Check sheet for the modelled part. Datum: model origin and axes. Units: mm. Face numbers are marked on the shaded views. A direction names the side the tool comes from. Give positions to 0.01 mm unless a question says otherwise; leave off trailing zeros. Write each loop counter-clockwise with the first axis right and the second up, starting at its lowest first coordinate (ties: lowest second). Pieces come first, ordered by that corner, then holes. Notation, with made-up numbers: (-16.5, 43) -> (10.5, 43) arc R38 cw to (10.5, 82) -> close; hole circle Ø6 at (29.25, -2.5). An arc over 180 degrees is marked (long way). Use a Markdown table: item, result. Add a question column.
1. Cross-section at D-D (y = 32). Enter the section's corners in (x, z).
2. Cross-section at B-B (x = 73.5). Enter the section's corners in (y, z).
3. Scan lines: probe 1 along X at (y, z) = (23.5, -68); probe 2 along Y at (x, z) = (76, -69); probe 3 along Y at (x, z) = (64, -63). Record each from-to range of solid material in increasing order. Write a range as [from, to].
4. Cross-section at C-C (z = -65). Enter the section's corners in (x, y).
5. Cross-section at A-A (y = 58). Enter the section's corners in (x, z), then the cut area to 3 significant figures.
6. Gauge pin test, flat ends, axial feed: P1, Ø12, axis at x = 43, z = -59.5, coming from the +Y side; P2, Ø5, axis at x = 86, y = 21, coming from the +Z side; P3, Ø12.5, axis at x = 12.5, y = 51.5, coming from the -Z side. Record the tip position at first contact, or that the pin passes through.
7. Set-up check for the marked faces 1, 2, 3 and 4: record each of +Z, -Z, +X, -X, +Y, -Y from which the full face is reachable in a straight line by a thin tool's end or side.
8. Release check for a two-part mould opening along Y. For the marked faces 5, 6 and 7 record: released by +Y, released by -Y, zero draft, split by the parting line, or undercut.
from build123d import *

# Parameters (mm, degrees)
BOSS_EXTRUDE1_DEPTH = 40
SKETCH1_3_W         = 50
SKETCH1_3_H         = 40
BOSS_EXTRUDE2_DEPTH = 20
BOSS_EXTRUDE3_DEPTH = 65
SKETCH2_W           = 10
SKETCH2_H           = 41
CUT_EXTRUDE1_DEPTH  = 141.890028036


with BuildPart() as part:
    # Sketch1 → Boss-Extrude1 (new body)
    with BuildSketch(Plane(origin=(0, 0, 0), x_dir=(1, 0, 0), z_dir=(0, 1, 0))):
        Polygon((0, 75), (0, 25), (30, 25), (30, 10), (70, 10), (70, 25), (100, 25), (100, 75), (75, 75), (75, 35), (25, 35), (25, 75), align=None)
    extrude(amount=BOSS_EXTRUDE1_DEPTH)

    # Sketch1_3 → Boss-Extrude2 (add)
    with BuildSketch(Plane(origin=(0, 0, 0), x_dir=(1, 0, 0), z_dir=(0, 1, 0))):
        with Locations((50, 55)):
            Rectangle(SKETCH1_3_W, SKETCH1_3_H)
    extrude(amount=BOSS_EXTRUDE2_DEPTH)

    # Sketch1_4 → Boss-Extrude3 (add)
    with BuildSketch(Plane(origin=(0, 0, 0), x_dir=(1, 0, 0), z_dir=(0, 1, 0))):
        Polygon((70, 25), (70, 10), (70, 0), (100, 0), (100, 25), align=None)
        Polygon((0, 25), (0, 0), (30, 0), (30, 10), (30, 25), align=None)
    extrude(amount=BOSS_EXTRUDE3_DEPTH)

    # Sketch2 → Cut-Extrude1 (cut, through all)
    with BuildSketch(Plane(origin=(100, 0, 0), x_dir=(0, 0, -1), z_dir=(1, 0, 0))):
        with Locations((5, 32.5)):
            Rectangle(SKETCH2_W, SKETCH2_H)
    extrude(amount=-CUT_EXTRUDE1_DEPTH, mode=Mode.SUBTRACT)


solid = part.part
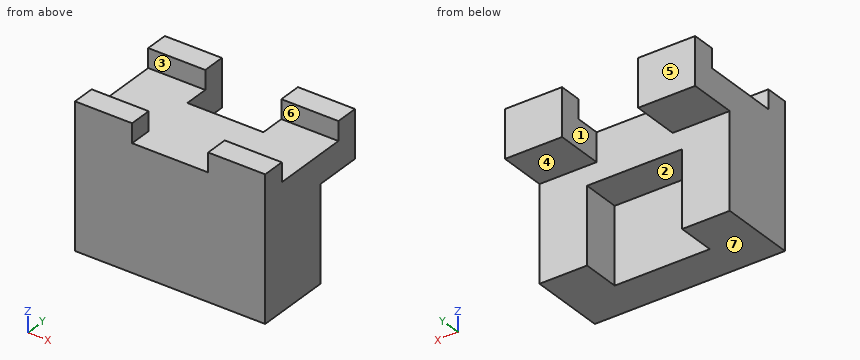
Worked answers:
| question | item | result |
|---|---|---|
| 1 | outline | (0, -75) -> (25, -75) -> (25, -35) -> (75, -35) -> (75, -75) -> (100, -75) -> (100, -10) -> (0, -10) -> close |
| 2 | outline | (0, -75) -> (20, -75) -> (20, -35) -> (40, -35) -> (40, -25) -> (65, -25) -> (65, 0) -> (53, 0) -> (53, -10) -> (12, -10) -> (12, 0) -> (0, 0) -> close |
| 3 | probe 1 | x = [0, 25], [75, 100] |
| 3 | probe 2 | y = [0, 40] |
| 3 | probe 3 | y = [0, 20] |
| 4 | outline | (0, 0) -> (100, 0) -> (100, 40) -> (75, 40) -> (75, 20) -> (25, 20) -> (25, 40) -> (0, 40) -> close |
| 5 | outline | (0, -25) -> (30, -25) -> (30, 0) -> (0, 0) -> close; (70, -25) -> (100, -25) -> (100, 0) -> (70, 0) -> close |
| 5 | area | 1,500 mm² |
| 6 | P1 | stops at y = 20 |
| 6 | P2 | stops at z = -10 |
| 6 | P3 | stops at z = -25 |
| 7 | face 1 | +Z, -Z, +Y |
| 7 | face 2 | -Z, +Y |
| 7 | face 3 | +Z, +X, -X |
| 7 | face 4 | -Z, +X, -X, +Y |
| 8 | face 5 | released by +Y |
| 8 | face 6 | undercut |
| 8 | face 7 | zero draft |
